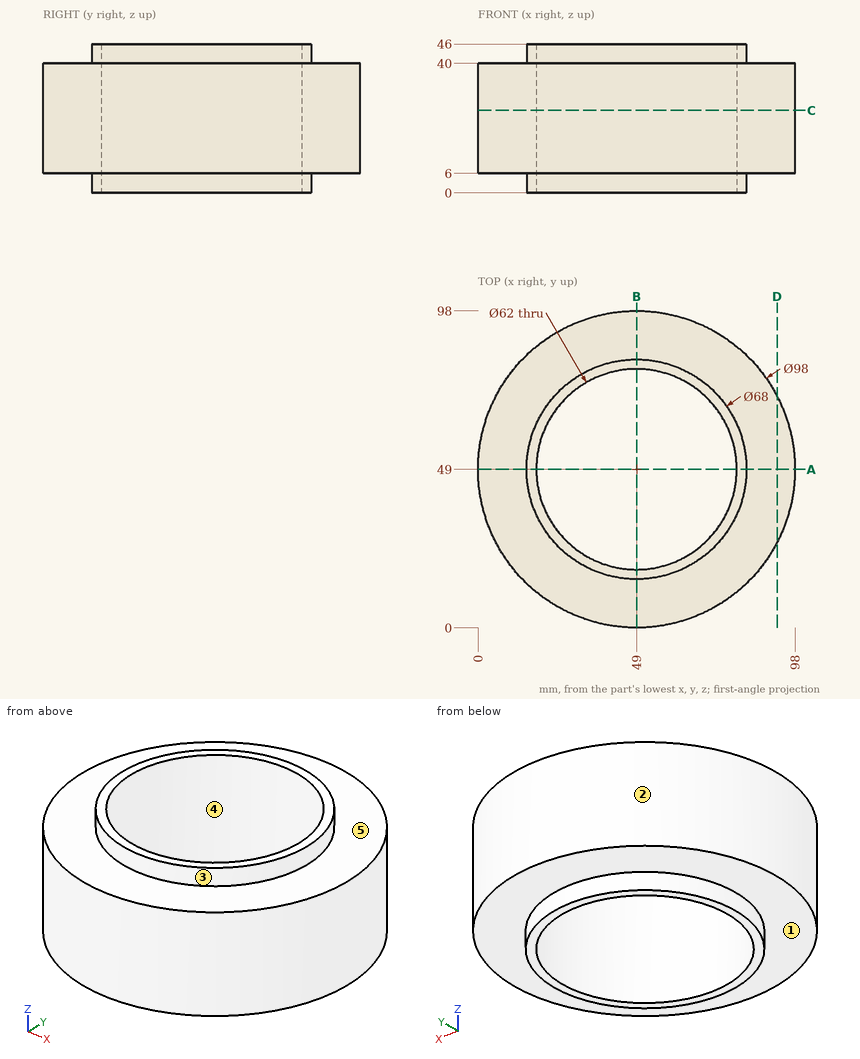
Job drawing, mm, ordinate dimensions from the low corner. One solid piece. A direction names the side the tool comes from. Give positions to 0.01 mm unless a question says otherwise; leave off trailing zeros. Loops run counter-clockwise (first coordinate to the right, second up) from the corner with the lowest first, then second, coordinate; pieces in that order, holes last. Notation, with made-up numbers: M 67.5,-32.5 L 107.5,-32.5 A9 cw 107.5,-20.5 Z; hole C 72.5,19 d1. An arc over 180 degrees is marked long. Answer in a Markdown table with one row per item. Add a question column.
Item 1: Mould opens along X. For the marked faces 3, 4 and 5 say: +X half, -X half, draft (parallel to the pull), parting line (faces both ways), or undercut.
Item 2: Probe probe 1 along Y at (x, z) = (49, 22); probe 2 along X at (y, z) = (50, 17.5); probe 3 along Z at (x, y) = (12, 76). List the from-to ranges inside material, lowest first.
Item 3: Band-saw the part on C-C on z = 25.5. Give the cut face in (x, y).
Item 4: Band-saw the part on A-A on y = 49. Give the cut face in (x, z).
Item 5: Drop flat-ended pins along their axis: P1, Ø3, axis at y = 14.5, z = 13, coming from the +X side; P2, Ø5, axis at y = 40, z = 34.5, coming from the -X side; P3, Ø1.5, axis at y = 77, z = 28.5, coming from the -X side. Give the stop position or say it passes through.
Item 6: Tool access for the marked faces 1 and 2: list every direction of +Z, -Z, +X, -X, +Y, -Y with a clear straight run to the whole face (end or side of a thin tool).
Item 7: Band-saw the part on D-D on x = 92.5. Give the cut face in (y, z).
Reply:
| question | item | result |
|---|---|---|
| 1 | face 3 | parting line |
| 1 | face 4 | undercut |
| 1 | face 5 | draft |
| 2 | probe 1 | y = 0 to 18, 80 to 98 |
| 2 | probe 2 | x = 0.01 to 18.02, 79.98 to 97.99 |
| 2 | probe 3 | z = 6 to 40 |
| 3 | outline | C 49,49 d98; hole C 49,49 d62 |
| 4 | outline | M 0,6 L 15,6 L 15,0 L 18,0 L 18,46 L 15,46 L 15,40 L 0,40 Z; M 80,0 L 83,0 L 83,6 L 98,6 L 98,40 L 83,40 L 83,46 L 80,46 Z |
| 5 | P1 | stops at x = 85.22 |
| 5 | P2 | stops at x = 0.43 |
| 5 | P3 | stops at x = 8.28 |
| 6 | face 1 | -Z |
| 6 | face 2 | +Z, -Z |
| 7 | outline | M 26.44,6 L 71.56,6 L 71.56,40 L 26.44,40 Z |
